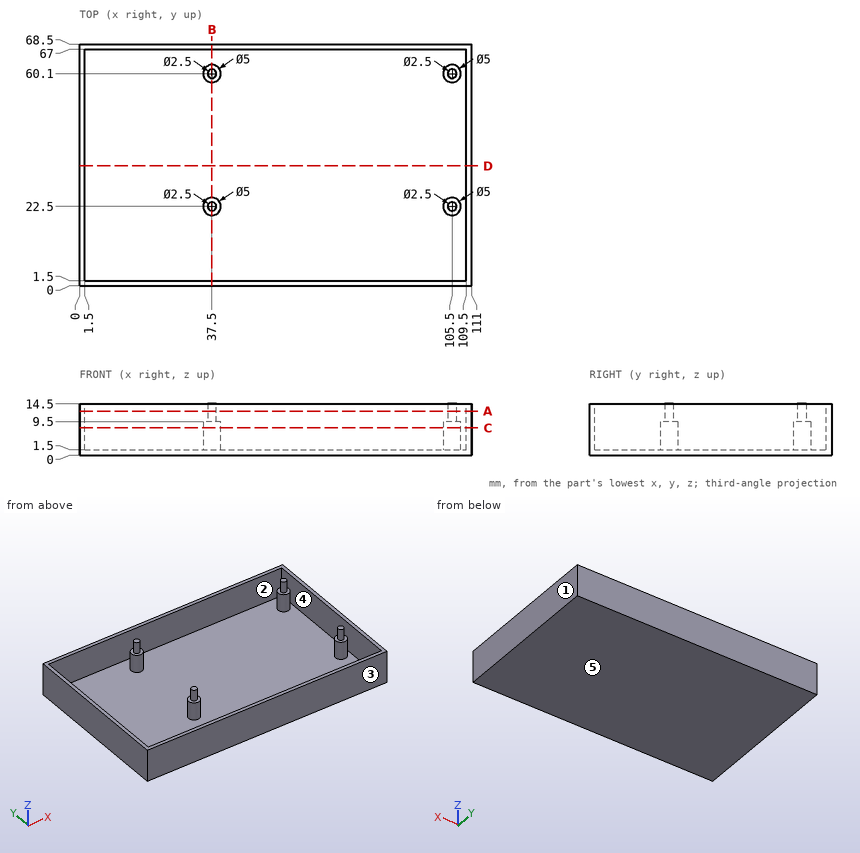
Design review of the part shown in the three views and the two pictorial views. Dimensions are in mm from the part's minimum x, y and z. A direction names the side the tool comes from. Round coordinates to 2 decimals unless told otherwise and drop trailing zeros. Loops run counter-clockwise (first coordinate to the right, second up) from the corner with the lowest first, then second, coordinate; pieces in that order, holes last. Notation, with made-up numbers: M 72,74 L 85,74 A23 ccw 85,84 Z; hole C 2.5,13.5 d9. An arc over 180 degrees is marked long. Put each result on its own line as item: value.
Q1. To check wall thickness, follow L1, parallel to Y at x = 105.5, z = 7; L2, parallel to X at y = 35, z = 2; L3, parallel to Y at x = 100, z = 2. State the ranges of each line that lie inside material, in increasing order.
Result set:
L1: y = 0 to 1.5, 20 to 25, 57.6 to 62.6, 67 to 68.5
L2: x = 0 to 1.5, 109.5 to 111
L3: y = 0 to 1.5, 67 to 68.5
Q2. Consider section B-B, the plane x = 37.5. Give the boundary of the cut face in (y, z).
Result set:
outline: M 0,0 L 68.5,0 L 68.5,14.5 L 67,14.5 L 67,1.5 L 62.6,1.5 L 62.6,9.5 L 61.35,9.5 L 61.35,14.5 L 58.85,14.5 L 58.85,9.5 L 57.6,9.5 L 57.6,1.5 L 25,1.5 L 25,9.5 L 23.75,9.5 L 23.75,14.5 L 21.25,14.5 L 21.25,9.5 L 20,9.5 L 20,1.5 L 1.5,1.5 L 1.5,14.5 L 0,14.5 Z
Q3. Consider section A-A, the plane z = 12.5. Give the boundary of the cut face in (x, y).
Result set:
outline: M 0,0 L 111,0 L 111,68.5 L 0,68.5 Z; C 37.5,22.5 d2.5; C 37.5,60.1 d2.5; C 105.5,22.5 d2.5; C 105.5,60.1 d2.5; hole M 1.5,1.5 L 109.5,1.5 L 109.5,67 L 1.5,67 Z
Q4. Consider section D-D, the plane y = 34. Give the boundary of the cut face in (x, z), then the cut area to 4 significant figures.
Result set:
outline: M 0,0 L 111,0 L 111,14.5 L 109.5,14.5 L 109.5,1.5 L 1.5,1.5 L 1.5,14.5 L 0,14.5 Z
area: 205.5 mm²
Q5. Mouldability with a two-part tool opening along X and no side actions: class the marked faces 1, 2 and 3 as released by +X, released by -X, zero draft, split by the parting line, or undercut.
Result set:
face 1: released by +X
face 2: undercut
face 3: zero draft
Q6. Consider section C-C, the plane z = 7.75. Give the boundary of the cut face in (x, y).
Result set:
outline: M 0,0 L 111,0 L 111,68.5 L 0,68.5 Z; C 37.5,22.5 d5; C 37.5,60.1 d5; C 105.5,22.5 d5; C 105.5,60.1 d5; hole M 1.5,1.5 L 109.5,1.5 L 109.5,67 L 1.5,67 Z
Q7. For pin 1 (6 mm diameter, centred on x = 54, y = 16.5, fed in from +Z), flat-tipped, find the tip position at first contact; note if it passes through.
Result set:
pin 1: stops at z = 1.5
Q8. Machinability: for the marked faces 4 and 5, which of the approach directions +Z, -Z, +X, -X, +Y, -Y give a long, thin tool a straight path to every point of the face, cutting with its end or side? Answer none if there is none.
Result set:
face 4: +Z
face 5: -Z, +X, -X, +Y, -Y
